The drawing under review shows one solid part. Ordinate dimensions are in mm from its lowest x, y, z. Round coordinates to 2 decimals unless told otherwise and drop trailing zeros. Write each loop counter-clockwise with the first axis right and the second up, starting at its lowest first coordinate (ties: lowest second). Pieces come first, ordered by that corner, then holes.
Item 1: Add section A-A (y = 6.35). Give the boundary of the cut face in (x, z) (1 decimal).
Item 2: Add section B-B (y = 62). Give the boundary of the cut face in (x, z).
Item 3: Add section D-D (y = 25). Give the boundary of the cut face in (x, z) (1 decimal).
Item 4: Add section C-C (x = 128). Give the boundary of the cut face in (y, z).
Item 5: To check wall thickness, follow L1, parallel to X at y = 55, z = 9.25; L2, parallel to Y at x = 86, z = 7 (1 decimal); L3, parallel to Y at x = 75, z = 11.5. State the ranges of each line that lie inside material, in increasing order.
Item 6: Draft analysis for pull direction X (two halves, no side actions). For the marked faces 1, 2, 3 and 4, state which applies: +X half, -X half, draft (parallel to the pull), parting line (faces both ways), or undercut.
Item 7: Clearance check with flat-ended pins moving along their axes: pin 1 Ø4 at (y, z) = (14.5, 3) entering from -X (1 decimal); pin 2 Ø0.9 at (x, z) = (80.5, 14.5) entering from -Y; pin 3 Ø5 at (x, z) = (107.5, 14) entering from +Y. State where each tip first meets the part, or that it passes through.
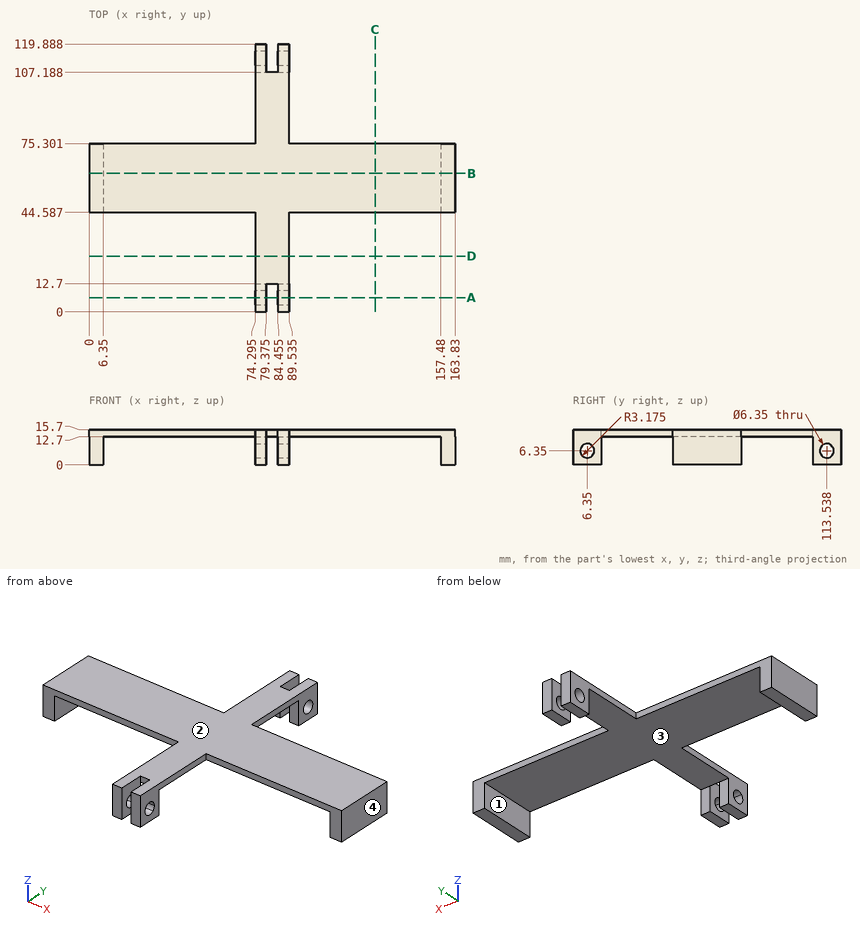
Numbers:
1. outline: (74.3, 0) - (79.4, 0) - (79.4, 3.2) - (74.3, 3.2) - close; (74.3, 9.5) - (79.4, 9.5) - (79.4, 15.7) - (74.3, 15.7) - close; (84.5, 0) - (89.5, 0) - (89.5, 3.2) - (84.5, 3.2) - close; (84.5, 9.5) - (89.5, 9.5) - (89.5, 15.7) - (84.5, 15.7) - close
2. outline: (0, 0) - (6.35, 0) - (6.35, 12.7) - (157.48, 12.7) - (157.48, 0) - (163.83, 0) - (163.83, 15.7) - (0, 15.7) - close
3. outline: (74.3, 12.7) - (89.5, 12.7) - (89.5, 15.7) - (74.3, 15.7) - close
4. outline: (44.59, 12.7) - (75.3, 12.7) - (75.3, 15.7) - (44.59, 15.7) - close
5. L1: x = 0 to 6.35, 157.48 to 163.83
5. L2: y = 0 to 3.2, 9.5 to 12.7, 107.2 to 110.4, 116.6 to 119.9
5. L3: y = 0 to 12.7, 107.19 to 119.89
6. face 1: undercut
6. face 2: draft
6. face 3: undercut
6. face 4: +X half
7. pin 1: stops at x = 74.3
7. pin 2: stops at y = 12.7
7. pin 3: stops at y = 75.3
